from build123d import *

# Parameters (mm, degrees)
F0_W     = 106
F0_H     = 127
F1_DEPTH = 44.4
F2_R     = 9
F3_DEPTH = 22.5
F2_R_2   = 5
F4_DEPTH = 26.6


with BuildPart() as f1:
    # F0 (on Top) → F1 (new body)
    with BuildSketch(Plane.XY):
        with Locations((-53, 63.5)):
            Rectangle(F0_W, F0_H)
    extrude(amount=F1_DEPTH)

    # F2 (on face) → F3 (join)
    with BuildSketch(Plane(origin=(-106, 0, 0), x_dir=(0, -1, 0), z_dir=(-1, 0, 0))):
        with Locations((-109, 22.2)):
            Circle(F2_R)
    extrude(amount=F3_DEPTH)

    # F2 (on face) → F4 (join)
    with BuildSketch(Plane(origin=(-106, 0, 0), x_dir=(0, -1, 0), z_dir=(-1, 0, 0))):
        with Locations((-8, 22.2)):
            Circle(F2_R_2)
    extrude(amount=F4_DEPTH)


solid = f1.part
The listing builds one solid part. Answer for the finished solid, in the listing's coordinates (mm). A direction names the side the tool comes from. Coordinates: 2 decimals unless noted, no trailing zeros. Write each loop counter-clockwise with the first axis right and the second up, starting at its lowest first coordinate (ties: lowest second). Pieces come first, ordered by that corner, then holes. Notation, with made-up numbers: (76.25, 6) - (114.25, 6) arc R9 cw to (114.25, 15) - close; hole circle Ø1 at (-21, 83). An arc over 180 degrees is marked (long way). Put each result on its own line as item: value.
1. The part is cut by section A-A on y = 109. Give the vertices of the cut face in (x, z).
Answer sheet:
outline: (-128.5, 13.2) - (-106, 13.2) - (-106, 0) - (0, 0) - (0, 44.4) - (-106, 44.4) - (-106, 31.2) - (-128.5, 31.2) - close
2. Determine the mould class of faces 4 (the face through (-54, 64, 44.4)), 5 (the face through (-119.11, 3.23, 23.7)), 6 (the face through (-54, 127, 22)), 7 (the face through (-106, 63, 22)) for opening direction Y: pulls with the +Y half, pulls with the -Y half, needs draft (parallel to the pull), parting line crosses it, or undercut.
Answer sheet:
face 4: needs draft
face 5: undercut
face 6: pulls with the +Y half
face 7: undercut
3. Flat-ended cylindrical pins translate along their axes: pin 1 Ø2 at (y, z) = (101, 15.5) entering from -X; pin 2 Ø8 at (x, z) = (-114, 6) entering from -Y; pin 3 Ø14.5 at (y, z) = (108, 23) entering from -X. Find the tip coordinate at first contact, or state that the pin passes through.
Answer sheet:
pin 1: stops at x = -106
pin 2: passes through
pin 3: stops at x = -128.5
4. Find the intervals of material crossed by line 1 along X through (y, z) = (48, 2.5); line 2 along X through (y, z) = (117, 21), in increasing order. Write a range as from..to.
Answer sheet:
line 1: x = -106..0
line 2: x = -128.5..0
5. A tool of negligible diameter and unlimited length cuts with its end or side. For faces 1 (the face through (-128.5, 109, 22)), 2 (the face through (-117.092, 100.416, 24.903)), 3 (the face through (0, 63, 22)), from which of +Z, -Z, +X, -X, +Y, -Y can it reach the whole face along a straight path? Write none if from no direction.
Answer sheet:
face 1: +Z, -Z, -X, +Y
face 2: -X
face 3: +Z, -Z, +X, +Y, -Y
6. The part is cut by section B-B on z = 22.2. Give the vertices of the cut face in (x, y).
Answer sheet:
outline: (-132.6, 3) - (-106, 3) - (-106, 0) - (0, 0) - (0, 127) - (-106, 127) - (-106, 118) - (-128.5, 118) - (-128.5, 100) - (-106, 100) - (-106, 13) - (-132.6, 13) - close
7. The part is cut by section C-C on y = 8. Give the vertices of the cut face in (x, z), plus the area to 3 significant figures.
Answer sheet:
outline: (-132.6, 17.2) - (-106, 17.2) - (-106, 0) - (0, 0) - (0, 44.4) - (-106, 44.4) - (-106, 27.2) - (-132.6, 27.2) - close
area: 4,970 mm^2
8. The part is cut by section D-D on z = 5. Give the vertices of the cut face in (x, y), plus the area to 3 significant figures.
Answer sheet:
outline: (-106, 0) - (0, 0) - (0, 127) - (-106, 127) - close
area: 13,500 mm^2
